Autodesk Fusion 360 part; units mm, degrees
sketch "shape" plane through (0, 0, 0) normal (0, 1, 0) x (1, 0, 0)
  line L0 (170.5738, 28.4165) -> (-42.7862, 28.4165)
  line L1 (-42.7862, 28.4165) -> (-42.7862, -100.0835)
  line L2 (170.5738, -100.0835) -> (170.5738, 28.4165)
  line L3 (-42.7862, -100.0835) -> (170.5738, -100.0835)
  line L4 (-42.7862, 28.4165) -> (-42.7862, 29.4165)
  line L5 (-42.7862, 28.4165) -> (-43.7862, 28.4165)
  line L6 (-42.7862, 28.4165) -> (-43.7862, 28.4165)
  line L7 (-43.7862, 28.4165) -> (-43.7862, 29.4165)
  line L8 (-43.7862, 29.4165) -> (-42.7862, 29.4165)
  line L9 (-42.7862, 29.4165) -> (-42.7862, 28.4165)
  line L10 (-43.7862, 29.4165) -> (171.5738, 29.4165)
  line L11 (171.5738, 29.4165) -> (171.5738, -101.0835)
  line L12 (171.5738, -101.0835) -> (-43.7862, -101.0835)
  line L13 (-43.7862, -101.0835) -> (-43.7862, 29.4165)
  dimension "d1" = 213.36
  dimension "d2" = 128.5
  dimension "d3" = 1
  dimension "d4" = 1
  dimension "d5" = 130.5
extrude "Extrude1" add sketch "shape" along normal blind 1 contours L0 L1 L2 L3
extrude "Extrude2" add sketch "shape" along normal blind 106
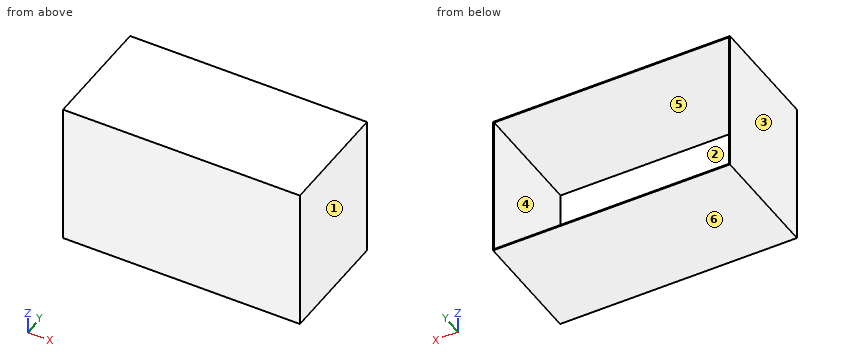
Input: part model. Units: mm. Frame: model coordinates. Face numbers are marked on the shaded views. A direction names the side the tool comes from. Give positions to 0.01 mm unless a question says otherwise; leave off trailing zeros. Loops run counter-clockwise (first coordinate to the right, second up) from the corner with the lowest first, then second, coordinate; pieces in that order, holes last. Notation, with made-up numbers: M 46.5,-27.75 L 56.5,-27.75 A19 cw 56.5,-1.75 Z; hole C 81,39.25 d9. An arc over 180 degrees is marked long. Use one line per item in the form item = value.
1. First-contact query: pin 1 (8 mm diameter, centred on x = 27, z = 74.5, fed in from +Y). Flat tip, straight axial feed; report the tip coordinate or a pass-through.
Numbers:
pin_1 = 1
2. Reachability of the marked faces 1 and 2 from +Z, -Z, +X, -X, +Y, -Y: full face, straight path, thin tool, end or side. Return the list, or none.
Numbers:
face_1 = +Z, -Z, +X, +Y, -Y
face_2 = +Y
3. Section query B-B, the plane x = 83.5. Return the cut outline in (y, z).
Numbers:
outline = M 0,-29.42 L 106,-29.42 L 106,-28.42 L 1,-28.42 L 1,100.08 L 106,100.08 L 106,101.08 L 0,101.08 Z
4. Line query: L1, parallel to Z at x = 72, y = 59.5; L2, parallel to X at y = 48, z = 94; L3, parallel to Y at x = -11.5, z = 17. Output: solid intervals per line, ascending.
Numbers:
L1 = -29.42 to -28.42, 100.08 to 101.08
L2 = -43.79 to -42.79, 170.57 to 171.57
L3 = 0 to 1
5. Section query C-C, the plane y = 12. Return the cut outline in (x, z), and give its area (3 significant figures).
Numbers:
outline = M -43.79,-29.42 L 171.57,-29.42 L 171.57,101.08 L -43.79,101.08 Z; hole M -42.79,-28.42 L 170.57,-28.42 L 170.57,100.08 L -42.79,100.08 Z
area = 688 mm²
6. Section query A-A, the plane z = -4.5. Return the cut outline in (x, y), and give its area (3 significant figures).
Numbers:
outline = M -43.79,0 L 171.57,0 L 171.57,106 L 170.57,106 L 170.57,1 L -42.79,1 L -42.79,106 L -43.79,106 Z
area = 425 mm²
7. Pull-direction query (Z, two-part tool) for the marked faces 3, 4, 5 and 6; classes: released by +Z, released by -Z, zero draft, split by the parting line, or undercut.
Numbers:
face_3 = zero draft
face_4 = undercut
face_5 = undercut
face_6 = released by -Z
